Check sheet for the drawn part. Datum: minimum x, y, z corner. Units: mm. A direction names the side the tool comes from. Coordinates: 2 decimals unless noted, no trailing zeros. Write each loop counter-clockwise with the first axis right and the second up, starting at its lowest first coordinate (ties: lowest second). Pieces come first, ordered by that corner, then holes. Notation, with made-up numbers: (-6.5, 44) -> (37.5, 44) arc R18 ccw to (37.5, 62) -> close; hole circle Ø2 at (77.5, -26). An arc over 180 degrees is marked (long way). Write item = value, one per line. Start each with the question number.
(1) Material ranges on probe 1 along Y at (x, z) = (101.6, 15.5); probe 2 along Z at (x, y) = (123, 24); probe 3 along X at (y, z) = (190, 15), recorded low to high. Write a range as [from, to].
(2) Section check B-B (y = 190.5). Record the cut outline in (x, z).
(3) Gauge pin test, flat ends, axial feed: pin 1 Ø6 at (x, y) = (51.5, 57) entering from -Z; pin 2 Ø4 at (x, z) = (39, 125) entering from -Y; pin 3 Ø8 at (x, z) = (46.5, 23) entering from +Y (1 decimal). Record the tip position at first contact, or that the pin passes through.
(4) Section check A-A (y = 101.6). Record the cut outline in (x, z) (1 decimal), plus the area to 3 significant figures.
(5) Section check C-C (z = 21.5). Record the cut outline in (x, y).
(6) Set-up check for the marked faces 1 and 2: record each of +Z, -Z, +X, -X, +Y, -Y from which the full face is reachable in a straight line by a thin tool's end or side.
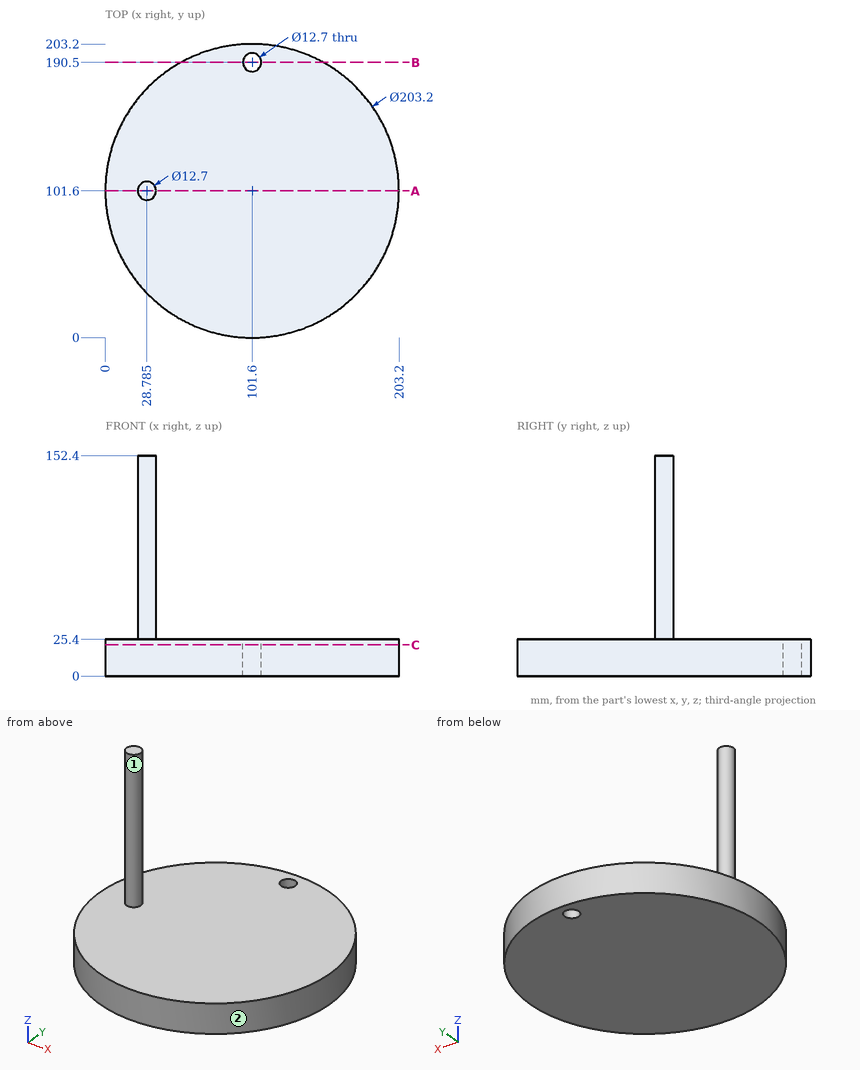
Response:
q1.probe_1 = [0, 184.15], [196.85, 203.2]
q1.probe_2 = [0, 25.4]
q1.probe_3 = [51.52, 95.27], [107.93, 151.68]
q2.outline = (52.41, 0) -> (95.25, 0) -> (95.25, 25.4) -> (52.41, 25.4) -> close; (107.95, 0) -> (150.79, 0) -> (150.79, 25.4) -> (107.95, 25.4) -> close
q3.pin_1 = 0
q3.pin_2 = through
q3.pin_3 = 189.4
q4.outline = (0, 0) -> (203.2, 0) -> (203.2, 25.4) -> (35.1, 25.4) -> (35.1, 152.4) -> (22.4, 152.4) -> (22.4, 25.4) -> (0, 25.4) -> close
q4.area = 6,770 mm2
q5.outline = circle Ø203.2 at (101.6, 101.6); hole circle Ø12.7 at (101.6, 190.5)
q6.face_1 = +Z
q6.face_2 = +Z, -Z
